Verification items for the finished model (mm, model axes). A direction names the side the tool comes from. Round coordinates to 2 decimals unless told otherwise and drop trailing zeros. Order: outer loops, then holes, each group sorted by start corner. A loop starts at its lowest first (then second) coordinate and runs counter-clockwise, first axis right, second up. Notation, with made-up numbers: M 27.5,42.5 L 37.5,42.5 A14 ccw 37.5,68.5 Z; hole C 2,26.5 d7. An arc over 180 degrees is marked long. Use CSV: the item, a comma, the result in double quotes. Start each with the question number.
Q1. Sectioned sample at C-C (x = 350). Enter the section's corners in (y, z), and give its area (3 significant figures).
Q2. Sectioned sample at B-B (z = -178). Enter the section's corners in (x, y).
Q3. Sectioned sample at A-A (y = 161). Enter the section's corners in (x, z), and give its area (3 significant figures).
Q4. Scan lines: line 1 (X direction, y = 64.5, z = -812.5); line 2 (X direction, y = 27, z = -582); line 3 (Y direction, x = 809.5, z = -713.5). Record each from-to range of solid material in increasing order.
Q5. Gauge pin test, flat ends, axial feed: pin 1 Ø2 at (x, z) = (369, -591.5) entering from +Y; pin 2 Ø1.5 at (x, z) = (680.5, -592.5) entering from +Y; pin 3 Ø12 at (x, z) = (321.5, -644.5) entering from -Y. Record the tip position at first contact, or that the pin passes through.
Q6. Sectioned sample at D-D (z = -789). Enter the section's corners in (x, y).
Q7. Set-up check for faces 3 (the face through (217.33, 91.74, -450.8)), 4 (the face through (640.866, 90.145, -450.799)): record each of +Z, -Z, +X, -X, +Y, -Y from which the full face is reachable in a straight line by a thin tool's end or side.
Q8. Mould release check, pull along Z, two halves, no side actions. Record for faces 1 (the face through (211.619, 87.655, -450.799)), 2 (the face through (232, 97, -50.8)): +Z half, -Z half, draft (parallel to the pull), parting line (faces both ways), or undercut.
```python
from build123d import *

# Parameters (mm, degrees)
F1_DEPTH = 914.4
F4_DEPTH = 178.052639


with BuildPart() as f1:
    # F0 (on Top) → F1 (new body)
    with BuildSketch(Plane.XY):
        Polygon((-0.60751, 1.466659), (0, 0), (429.247171, 177.8), (858.494343, 0), (859.101853, 1.466659), (429.247171, 179.518298), align=None)
    extrude(amount=-F1_DEPTH)

    # F3 (on face) → F4 (cut, through all)
    with BuildSketch(Plane(origin=(0, 1.466659, 0), x_dir=(-1, 0, 0), z_dir=(0, 1, 0))):
        Polygon((-810.162893, -406.4), (-48.93896, -76.2), (-48.93896, -50.8), (-416.229916, -50.8), (-416.229916, -228.6), (-812.689867, -400.574461), align=None)
    extrude(amount=F4_DEPTH, mode=Mode.SUBTRACT)


solid = f1.part
```
Verdict:
1,outline,"M 144.97,-914.4 L 146.69,-914.4 L 146.69,-206.79 L 144.97,-206.79 Z; M 144.97,-50.8 L 146.69,-50.8 L 146.69,0 L 144.97,0 Z"
1,area,"1,300 mm²"
2,outline,"M -0.61,1.47 L 0,0 L 283.62,117.48 L 283.62,119.2 Z; M 416.23,172.41 L 429.25,177.8 L 858.49,0 L 859.1,1.47 L 429.25,179.52 L 416.23,174.13 Z"
3,outline,"M 384.54,-914.4 L 388.69,-914.4 L 388.69,-223.57 L 384.54,-221.78 Z; M 384.54,-50.8 L 388.69,-50.8 L 388.69,0 L 384.54,0 Z; M 469.81,-914.4 L 473.95,-914.4 L 473.95,-260.56 L 469.81,-258.76 Z; M 469.81,-251.84 L 473.95,-253.64 L 473.95,0 L 469.81,0 Z"
3,area,"6,840 mm²"
4,line 1,"x = 151.57 to 155.72, 702.78 to 706.93"
4,line 2,"x = 61.04 to 65.18, 793.31 to 797.46"
4,line 3,"y = 20.29 to 22.01"
5,pin 1,"stops at y = 154.98"
5,pin 2,"stops at y = 75.76"
5,pin 3,"stops at y = 130.68"
6,outline,"M -0.61,1.47 L 0,0 L 429.25,177.8 L 858.49,0 L 859.1,1.47 L 429.25,179.52 Z"
7,face 3,"+Z, -Z, -X, +Y"
7,face 4,"+Z, -Z, -Y"
8,face 1,"draft"
8,face 2,"undercut"
